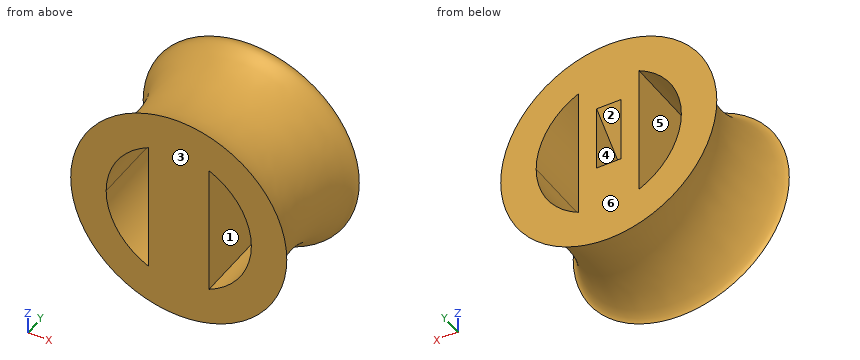
```python
from build123d import *

# Parameters (mm, degrees)
SKETCH2_R               = 9
BOSS_EXTRUDE1_DEPTH     = 10
CUT_EXTRUDE1_DEPTH      = 11.0000001
CUT_EXTRUDE2_DEPTH      = 1
CUT_EXTRUDE2_DEPTH_BACK = 1


with BuildPart() as part:
    # Sketch2 → Boss-Extrude1 (new body)
    with BuildSketch(Plane(origin=(0, 0, 0), x_dir=(1, 0, 0), z_dir=(0, 1, 0))):
        Circle(SKETCH2_R)
    extrude(amount=BOSS_EXTRUDE1_DEPTH)

    # Sketch3 → Cut-Revolve1 (revolve, cut)
    with BuildSketch(Plane.XY):
        with BuildLine():
            Line((-9, 10), (-9, 0))
            add(Edge.make_bspline(
                [(-9, 10), (-8.339177008, 10.090505936), (-6.320822992, 5), (-8.339177008, -0.090505936), (-9, 0)],
                knots=[0, 0, 0, 0, 0.256608512, 0.513217025, 0.513217025, 0.513217025, 0.513217025], degree=3))
        make_face()
    revolve(axis=Axis((0, 0, 0), (0, 1, 0)), mode=Mode.SUBTRACT)

    # Sketch4 → Cut-Extrude1 (cut, through all)
    with BuildSketch(Plane(origin=(0, 10, 0), x_dir=(1, 0, 0), z_dir=(0, 1, 0))):
        with BuildLine():
            ThreePointArc((-6, 0), (-5.049752469, -3.240370349), (-2.5, -5.454356057))
            Line((-2.5, -5.454356057), (-2.5, 0))
            Line((-2.5, 0), (-6, 0))
        make_face()
        with BuildLine():
            Line((-6, 0), (-2.5, 0))
            Line((-2.5, 0), (-2.5, 5.454356057))
            ThreePointArc((-2.5, 5.454356057), (-5.049752469, 3.240370349), (-6, 0))
        make_face()
        with BuildLine():
            Line((2.5, 0), (2.5, -5.454356057))
            ThreePointArc((2.5, -5.454356057), (5.049752469, -3.240370349), (6, 0))
            Line((6, 0), (2.5, 0))
        make_face()
        with BuildLine():
            Line((2.5, 5.454356057), (2.5, 0))
            Line((2.5, 0), (6, 0))
            ThreePointArc((6, 0), (5.049752469, 3.240370349), (2.5, 5.454356057))
        make_face()
    extrude(amount=-CUT_EXTRUDE1_DEPTH, mode=Mode.SUBTRACT)

    # Sketch5 → Cut-Extrude2 (cut, two sides)
    with BuildSketch(Plane.ZY) as cut_extrude2_sk:
        with BuildLine():
            Line((-2.01113744, 10), (-4.520166387, 7.276604619))
            ThreePointArc((-4.520166387, 7.276604619), (-4.783869038, 6.55810107), (-4.462276239, 5.863576406))
            Line((-4.462276239, 5.863576406), (-2.991357878, 4.508438341))
            ThreePointArc((-2.991357878, 4.508438341), (-2.272854329, 4.24473569), (-1.578329665, 4.566328489))
            Line((-1.578329665, 4.566328489), (3.427641633, 10))
            Line((3.427641633, 10), (-2.01113744, 10))
        make_face()
    extrude(amount=CUT_EXTRUDE2_DEPTH, mode=Mode.SUBTRACT)
    extrude(cut_extrude2_sk.sketch, amount=-CUT_EXTRUDE2_DEPTH_BACK, mode=Mode.SUBTRACT)


solid = part.part
```
Geometry check sheet. Reference: the model listing, model coordinates, mm. Face numbers are marked on the shaded views. A direction names the side the tool comes from. Round coordinates to 2 decimals unless told otherwise and drop trailing zeros. Use a Markdown table: item, result.
(1) Mould release check, pull along Y, two halves, no side actions. Record for the marked faces 4, 5 and 6: released by +Y, released by -Y, zero draft, split by the parting line, or undercut.
Calculated:
| item | result |
|---|---|
| face 4 | undercut |
| face 5 | zero draft |
| face 6 | released by +Y |
(2) Go/stop test with flat-tipped pins: P1, Ø3, axis at y = 5, z = -1.5, coming from the +X side; P2, Ø2, axis at x = -4.5, y = 2, coming from the +Z side; P3, Ø5, axis at y = 2.5, z = 6, coming from the -X side. Record where each tip stops, or that it passes through.
Calculated:
| item | result |
|---|---|
| P1 | x = 7.38 |
| P2 | z = 7.05 |
| P3 | x = -7.08 |
(3) Sectioned sample at A-A (z = -3.25). Give the number of separate pieces and of enclosed holes in the cut face, then the cut area to 3 significant figures.
Calculated:
| item | result |
|---|---|
| separate pieces | 3 |
| enclosed holes | 1 |
| area | 82.0 mm² |
(4) Set-up check for the marked faces 1, 2 and 3: record each of +Z, -Z, +X, -X, +Y, -Y from which the full face is reachable in a straight line by a thin tool's end or side.
Calculated:
| item | result |
|---|---|
| face 1 | +Y, -Y |
| face 2 | +Y |
| face 3 | +Z, -Z, +X, -X, -Y |
(5) Scan lines: probe 1 along X at (y, z) = (6, 1); probe 2 along X at (y, z) = (5, -1.75); probe 3 along X at (y, z) = (9.5, -1.5). Record each from-to range of solid material in increasing order.
Calculated:
| item | result |
|---|---|
| probe 1 | -7.31 to -5.92, -2.5 to 2.5, 5.92 to 7.31 |
| probe 2 | -7.12 to -5.74, -2.5 to -1, 1 to 2.5, 5.74 to 7.12 |
| probe 3 | -8.25 to -5.81, -2.5 to -1, 1 to 2.5, 5.81 to 8.25 |
